from build123d import *

# Parameters (mm, degrees)
SKETCH1_W          = 39.624
SKETCH1_H          = 7.366
PEEK_DEPTH         = 1.4224
SKETCH2_R          = 0.75
CUT_EXTRUDE1_DEPTH = 2.4224


with BuildPart() as part:
    # Sketch1 → PEEK (new body)
    with BuildSketch(Plane.XY):
        Rectangle(SKETCH1_W, SKETCH1_H)
    extrude(amount=PEEK_DEPTH)

    # Sketch2 → Cut-Extrude1 (cut, through all)
    with BuildSketch(Plane(origin=(0, 0, 0), x_dir=(-1, 0, 0), z_dir=(0, 0, -1))):
        with Locations((-18, -1.885)):
            Circle(SKETCH2_R)
        with Locations((-14.4, -1.885)):
            Circle(SKETCH2_R)
        with Locations((-10.8, -1.885)):
            Circle(SKETCH2_R)
        with Locations((-7.2, -1.885)):
            Circle(SKETCH2_R)
        with Locations((-3.6, -1.885)):
            Circle(SKETCH2_R)
        with Locations((0, -1.885)):
            Circle(SKETCH2_R)
        with Locations((3.6, -1.885)):
            Circle(SKETCH2_R)
        with Locations((7.2, -1.885)):
            Circle(SKETCH2_R)
        with Locations((10.8, -1.885)):
            Circle(SKETCH2_R)
        with Locations((14.4, -1.885)):
            Circle(SKETCH2_R)
        with Locations((18, -1.885)):
            Circle(SKETCH2_R)
        with Locations((16.2, 1.885)):
            Circle(SKETCH2_R)
        with Locations((12.6, 1.885)):
            Circle(SKETCH2_R)
        with Locations((9, 1.885)):
            Circle(SKETCH2_R)
        with Locations((5.4, 1.885)):
            Circle(SKETCH2_R)
        with Locations((1.8, 1.885)):
            Circle(SKETCH2_R)
        with Locations((-1.8, 1.885)):
            Circle(SKETCH2_R)
        with Locations((-5.4, 1.885)):
            Circle(SKETCH2_R)
        with Locations((-9, 1.885)):
            Circle(SKETCH2_R)
        with Locations((-12.6, 1.885)):
            Circle(SKETCH2_R)
        with Locations((-16.2, 1.885)):
            Circle(SKETCH2_R)
    extrude(amount=-CUT_EXTRUDE1_DEPTH, mode=Mode.SUBTRACT)


solid = part.part
Geometry: final body of the model. Coordinates: model frame, mm. Coordinates: 2 decimals unless noted, no trailing zeros. Write each loop counter-clockwise with the first axis right and the second up, starting at its lowest first coordinate (ties: lowest second). Pieces come first, ordered by that corner, then holes. Notation, with made-up numbers: (48, 30) - (93, 30) arc R18 ccw to (93, 42) - close; hole circle Ø4 at (80.25, 7.5). An arc over 180 degrees is marked (long way). Return JSON: item names as keys, results as strings.
Item 1: Section query B-B (z = 1.15). Count the separate pieces of the cut face and the enclosed holes in it, and give its area (3 significant figures).
Completed:
{"separate pieces": "1", "enclosed holes": "21", "area": "255 mm2"}
Item 2: Pull-direction query (X, two-part tool) for faces 1 (the face through (0, 3.683, 1)), 2 (the face through (-19.812, 0, 1)), 3 (the face through (10.085, -1.66, 0.701)); classes: +X half, -X half, draft (parallel to the pull), parting line (faces both ways), or undercut.
Completed:
{"face 1": "draft", "face 2": "-X half", "face 3": "undercut"}
Item 3: Pin query (flat end, axial travel): pin 1 Ø1.4 at (x, y) = (10.8, -1.885) entering from +Z. Return the tip coordinate at first contact, or that it passes through.
Completed:
{"pin 1": "passes through"}
Item 4: Section query A-A (x = 7.2). Output: boundary loops of the cut face in (y, z) (3 decimals), and give its area (3 significant figures).
Completed:
{"outline": "(-3.683, 0) - (-2.635, 0) - (-2.635, 1.422) - (-3.683, 1.422) - close; (-1.135, 0) - (3.683, 0) - (3.683, 1.422) - (-1.135, 1.422) - close", "area": "8.34 mm2"}
Item 5: Line query: L1, parallel to Y at x = -1.8, z = 0.6 (3 decimals); L2, parallel to Y at x = 0, z = 0.95 (3 decimals). Output: solid intervals per line, ascending.
Completed:
{"L1": "y = -3.683 to 1.135, 2.635 to 3.683", "L2": "y = -3.683 to -2.635, -1.135 to 3.683"}
Item 6: Section query C-C (x = -7.5). Output: boundary loops of the cut face in (y, z), and give its area (3 significant figures).
Completed:
{"outline": "(-3.68, 0) - (-2.57, 0) - (-2.57, 1.42) - (-3.68, 1.42) - close; (-1.2, 0) - (3.68, 0) - (3.68, 1.42) - (-1.2, 1.42) - close", "area": "8.52 mm2"}
